```python
from build123d import *

# Parameters (mm, degrees)
BOX004_W     = 7
BOX004_H     = 10
BOX004_DEPTH = 8
BOX003_W     = 20.5
BOX003_H     = 27
BOX003_DEPTH = 1.6


with BuildPart() as cube004:
    # Box004 → Box004 (new body)
    with BuildSketch(Plane(origin=(0, 8, 1.6), x_dir=(1, 0, 0), z_dir=(0, 0, 1))):
        with Locations((3.5, 5)):
            Rectangle(BOX004_W, BOX004_H)
    extrude(amount=BOX004_DEPTH)


with BuildPart() as obj1:
    # Box003 → Box003 (new body)
    with BuildSketch(Plane.XY):
        with Locations((10.25, 13.5)):
            Rectangle(BOX003_W, BOX003_H)
    extrude(amount=BOX003_DEPTH)

    # Fusion001: union Cube004
    add(cube004.part)


with BuildPart() as obj1_1:
    # Fusion001 placement: moved
    add(obj1.part.moved(Location((24, -52.25, 7))))


solid = obj1_1.part
```
Part model, mm, in its own coordinate system. A direction names the side the tool comes from. Coordinates: 2 decimals unless noted, no trailing zeros. Write each loop counter-clockwise with the first axis right and the second up, starting at its lowest first coordinate (ties: lowest second). Pieces come first, ordered by that corner, then holes.
Item 1: Pin check, flat tips, straight feed: pin 1 (3.5 mm diameter, centred on x = 28, z = 13, fed in from -Y); pin 2 (2 mm diameter, centred on y = -29, z = 9.5, fed in from +X); pin 3 (2 mm diameter, centred on x = 36.5, y = -40.5, fed in from +Z). Stop position of each tip, or through.
Item 2: Slice it at C-C (z = 11.5). Write the cut outline in (x, y).
Item 3: Slice it at B-B (y = -41). Write the cut outline in (x, z), and give its area (3 significant figures).
Item 4: Slice it at A-A (x = 25.75). Write the cut outline in (y, z), and give its area (3 significant figures).
Item 5: Probe line 1 (Z direction, x = 39.75, y = -41); line 2 (Y direction, x = 27, z = 9.75); line 3 (X direction, y = -42, z = 16). List the from-to ranges inside material, lowest first.
Item 6: Which spindle directions (+Z, -Z, +X, -X, +Y, -Y) get a long thin tool onto all of the face, cutting with end or side? Do faces 1 (the face through (24, -39, 11)), 2 (the face through (31, -39, 13)), 3 (the face through (27, -34.25, 13)), 4 (the face through (27, -44.25, 13)). Say none if no direction does.
Item 7: Slice it at D-D (x = 35.5). Write the cut outline in (y, z).
Results found:
1. pin 1: stops at y = -44.25
1. pin 2: stops at x = 44.5
1. pin 3: stops at z = 8.6
2. outline: (24, -44.25) - (31, -44.25) - (31, -34.25) - (24, -34.25) - close
3. outline: (24, 7) - (44.5, 7) - (44.5, 8.6) - (31, 8.6) - (31, 16.6) - (24, 16.6) - close
3. area: 88.8 mm2
4. outline: (-52.25, 7) - (-25.25, 7) - (-25.25, 8.6) - (-34.25, 8.6) - (-34.25, 16.6) - (-44.25, 16.6) - (-44.25, 8.6) - (-52.25, 8.6) - close
4. area: 123 mm2
5. line 1: z = 7 to 8.6
5. line 2: y = -44.25 to -34.25
5. line 3: x = 24 to 31
6. face 1: +Z, -Z, -X, +Y, -Y
6. face 2: +Z, +X, +Y, -Y
6. face 3: +Z, +X, -X, +Y
6. face 4: +Z, +X, -X, -Y
7. outline: (-52.25, 7) - (-25.25, 7) - (-25.25, 8.6) - (-52.25, 8.6) - close
